Could you check a few things on this drawing? It's one solid part, dimensions in mm from its lowest x, y, z. Give positions to 0.01 mm unless a question says otherwise; leave off trailing zeros. Loops run counter-clockwise (first coordinate to the right, second up) from the corner with the lowest first, then second, coordinate; pieces in that order, holes last. Notation, with made-up numbers: M 8.5,89 L 42.5,89 A30 cw 42.5,112 Z; hole C 33.5,-29.75 d4. An arc over 180 degrees is marked long. Answer as CSV lines item,"result". Start each with the question number.
Item 1: I want a section at C-C on y = 19.5. List the corners of the cut face in (x, z) for me.
Item 2: I want a section at B-B on z = 3.3. List the corners of the cut face in (x, y) for me.
Item 3: If I drill on line 1 along X through (y, z) = (70, 2.2); line 2 along Y through (x, z) = (10, 1.75); line 3 along Y through (x, z) = (207.5, 4.25), over which ranges is the centre line in solid material (lowest first)? Write a range as from..to.
Item 4: I want a section at A-A on x = 230. List the corners of the cut face in (y, z) for me, plus the area to 3 significant figures.
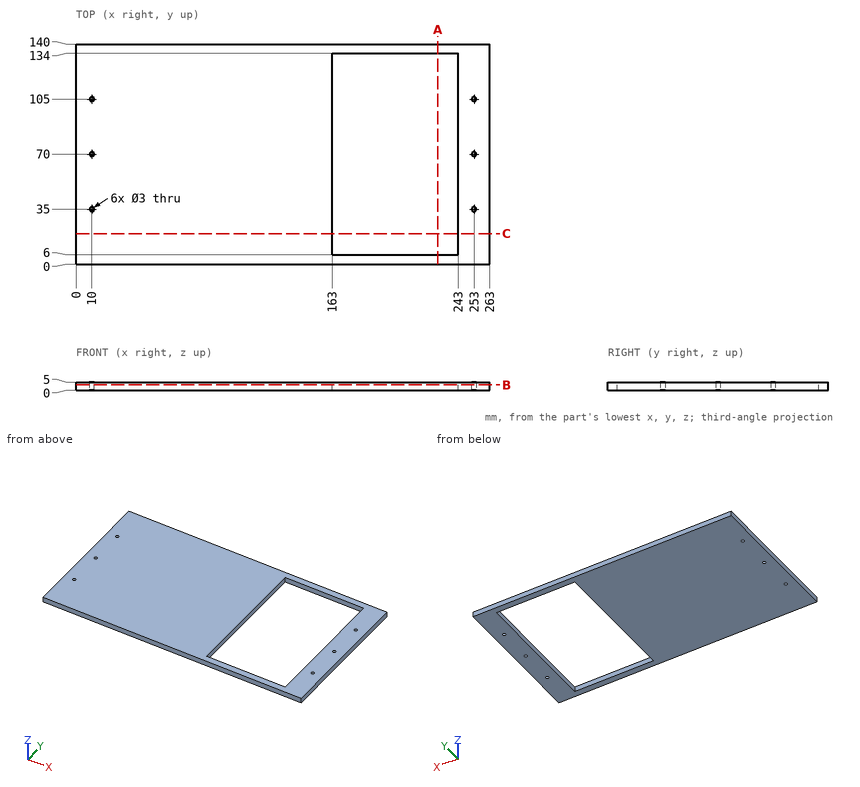
Result:
1,outline,"M 0,0 L 163,0 L 163,5 L 0,5 Z; M 243,0 L 263,0 L 263,5 L 243,5 Z"
2,outline,"M 0,0 L 263,0 L 263,140 L 0,140 Z; hole C 10,35 d3; hole C 10,70 d3; hole C 10,105 d3; hole M 163,6 L 243,6 L 243,134 L 163,134 Z; hole C 253,35 d3; hole C 253,70 d3; hole C 253,105 d3"
3,line 1,"0..8.5, 11.5..163, 243..251.5, 254.5..263"
3,line 2,"0..33.5, 36.5..68.5, 71.5..103.5, 106.5..140"
3,line 3,"0..6, 134..140"
4,outline,"M 0,0 L 6,0 L 6,5 L 0,5 Z; M 134,0 L 140,0 L 140,5 L 134,5 Z"
4,area,"60.0 mm^2"
